The model under review builds one solid part; all positions refer to its coordinate system, in mm. A direction names the side the tool comes from. Coordinates: 2 decimals unless noted, no trailing zeros. Write each loop counter-clockwise with the first axis right and the second up, starting at its lowest first coordinate (ties: lowest second). Pieces come first, ordered by that corner, then holes. Notation, with made-up numbers: (-9.75, 24.5) -> (10.25, 24.5) arc R25 cw to (10.25, 46.5) -> close; hole circle Ø7 at (43, 80). An arc over 180 degrees is marked (long way). Write each question's results on one line, items separated by ' | '.
```python
from build123d import *

# Parameters (mm, degrees)
F0_W     = 25.4
F0_H     = 82.55
F1_DEPTH = 38.1
F3_DEPTH = 76.2
F4_W     = 7.62
F4_H     = 10.16
F5_DEPTH = 25.4
F6_R     = 5.08


with BuildPart() as f1:
    # F0 (on Top) → F1 (new body)
    with BuildSketch(Plane.XY):
        with Locations((12.7, -41.275)):
            Rectangle(F0_W, F0_H)
    extrude(amount=F1_DEPTH)

    # F2 (on face) → F3 (cut)
    with BuildSketch(Plane.XY.offset(38.1)):
        with BuildLine():
            ThreePointArc((25.4, -1.677045), (34.697045, 7.62), (38.1, 20.32))
            ThreePointArc((38.1, 20.32), (0, 42.317045), (0, -1.677045))
            Line((0, -1.677045), (0, 0))
            Line((0, 0), (25.4, 0))
            Line((25.4, 0), (25.4, -1.677045))
        make_face()
        with BuildLine():
            Line((0, 0), (0, -1.677045))
            ThreePointArc((0, -1.677045), (12.7, -5.08), (25.4, -1.677045))
            Line((25.4, -1.677045), (25.4, 0))
            Line((25.4, 0), (0, 0))
        make_face()
    extrude(amount=-F3_DEPTH, mode=Mode.SUBTRACT)

    # F4 (on face) → F5 (cut)
    with BuildSketch(Plane.XY.offset(38.1)):
        with Locations((12.7, -17.78)):
            Rectangle(F4_W, F4_H)
    extrude(amount=-F5_DEPTH, mode=Mode.SUBTRACT)

    # F6
    f6_edges = [f1.edges().sort_by_distance(p)[0] for p in [
        (0, -42.113523, 38.1),
        (0, -42.113523, 0),
        (25.4, -42.113523, 38.1),
        (25.4, -42.113523, 0),
    ]]
    fillet(f6_edges, radius=F6_R)


solid = f1.part
```
Q1. Add section B-B (y = -20). Write out the cut boundary in (x, z), plus the area to 3 significant figures.
Solution:
outline: (0, 5.08) arc R5.08 ccw to (5.08, 0) -> (20.32, 0) arc R5.08 ccw to (25.4, 5.08) -> (25.4, 33.02) arc R5.08 ccw to (20.32, 38.1) -> (16.51, 38.1) -> (16.51, 12.7) -> (8.89, 12.7) -> (8.89, 38.1) -> (5.08, 38.1) arc R5.08 ccw to (0, 33.02) -> close | area: 752 mm²
Q2. Machinability: for faces 1 (the flat face through (8.89, -18, 26)), 2 (the cylindrical face through (1.449, -41.547, 1.528)), which of the approach directions +Z, -Z, +X, -X, +Y, -Y give a long, thin tool a straight path to every point of the face, cutting with its end or side? Answer none if there is none.
Solution:
face 1: +Z | face 2: -Z, -X, +Y, -Y
Q3. Add section A-A (z = 26). Write out the cut boundary in (x, y), plus the area to 3 significant figures.
Solution:
outline: (0, -82.55) -> (25.4, -82.55) -> (25.4, -1.68) arc R25.4 cw to (0, -1.68) -> close; hole (8.89, -22.86) -> (16.51, -22.86) -> (16.51, -12.7) -> (8.89, -12.7) -> close | area: 1,920 mm²
Q4. Draft analysis for pull direction X (two halves, no side actions). For faces 3 (the flat face through (0, -43, 19)), 4 (the flat face through (25.4, -43, 19)), 5 (the flat face through (13, -12.7, 26)), state which applies: pulls with the +X half, pulls with the -X half, needs draft (parallel to the pull), parting line crosses it, or undercut.
Solution:
face 3: pulls with the -X half | face 4: pulls with the +X half | face 5: undercut
Q5. For line 1 (X direction, y = -15.5, z = 33); line 2 (Y direction, x = 12.25, z = 15); line 3 (Z direction, x = 9.5, y = -21), list the stretches that pass through material, from the lowest coordinate up. Write a range as from..to.
Solution:
line 1: 0..8.89, 16.51..25.4 | line 2: -82.55..-22.86, -12.7..-5.08 | line 3: 0..12.7
Q6. Clearance check with flat-ended pins moving along their axes: P1, Ø8.5, axis at x = 12, z = 29.5, coming from the +Y side; P2, Ø2.5, axis at x = 11.5, y = -19.5, coming from the +Z side. State where each tip first meets the part, or that it passes through.
Solution:
P1: y = -4.59 | P2: z = 12.7
Q7. Add section D-D (y = -69.5). Write out the cut boundary in (x, z).
Solution:
outline: (0, 5.08) arc R5.08 ccw to (5.08, 0) -> (20.32, 0) arc R5.08 ccw to (25.4, 5.08) -> (25.4, 33.02) arc R5.08 ccw to (20.32, 38.1) -> (5.08, 38.1) arc R5.08 ccw to (0, 33.02) -> close
Q8. Add section C-C (x = 10.25). Write out the cut boundary in (y, z).
Solution:
outline: (-82.55, 0) -> (-4.96, 0) -> (-4.96, 38.1) -> (-12.7, 38.1) -> (-12.7, 12.7) -> (-22.86, 12.7) -> (-22.86, 38.1) -> (-82.55, 38.1) -> close
